Autodesk Inventor part; units mm, degrees
ref_plane "YZ Plane" through (0, 0, 0) normal (1, 0, 0) x (0, 1, 0)
ref_plane "XZ Plane" through (0, 0, 0) normal (0, 1, 0) x (-1, 0, 0)
ref_plane "XY Plane" through (0, 0, 0) normal (0, 0, 1) x (1, 0, 0)
sketch "Sketch1" plane through (0, 0, 0) normal (1, 0, 0) x (0, 1, 0)
  line L0 (0, 0) -> (25.4, 0)
  line L1 (25.4, 0) -> (25.4, -25.4)
  line L2 (25.4, -25.4) -> (0, -25.4)
  line L3 (0, -25.4) -> (0, 0)
  line L4 (23.8125, -1.5875) -> (1.5875, -1.5875)
  line L5 (1.5875, -1.5875) -> (1.5875, -23.8125)
  line L6 (1.5875, -23.8125) -> (23.8125, -23.8125)
  line L7 (23.8125, -23.8125) -> (23.8125, -1.5875)
  dimension "d0" = 25.4
  dimension "d1" = 25.4
  dimension "d2" = 1.5875
extrude "Extrusion1" add sketch "Sketch1" along normal blind 609.6
sketch "Sketch2" plane through (0, 25.4, 0) normal (0, 1, 0) x (1, 0, 0)
  line L0 (0, 1.5875) -> (0, 23.8125)
  line L1 (0, 12.7) -> (64.9449, 12.7) construction
  circle A0 centre (38.1, 12.7) radius 3.175
  circle A1 centre (63.5, 12.7) radius 3.175
  circle A2 centre (292.1, 12.7) radius 3.175
  point P0 (0, 0)
  dimension "d5" = 6.35
  dimension "d6" = 38.1
  dimension "d7" = 63.5
  dimension "d8" = 292.1
extrude "Extrusion2" cut sketch "Sketch2" against normal blind 25.4
sketch "Sketch3" plane through (0, 0, 0) normal (0, 0, 1) x (1, 0, 0)
  line L0 (0, 23.8125) -> (0, 1.5875)
  line L1 (0, 12.7) -> (84.2174, 12.7) construction
  circle A0 centre (241.3, 12.7) radius 3.175
  point P0 (0, 0)
  dimension "d11" = 6.35
  dimension "d12" = 241.3
extrude "Extrusion3" cut sketch "Sketch3" against normal blind 25.4
properties part number "Short horizontal"
Geometry: final body of the model. Coordinates: model frame, mm. A direction names the side the tool comes from. Coordinates: 2 decimals unless noted, no trailing zeros. Loops run counter-clockwise (first coordinate to the right, second up) from the corner with the lowest first, then second, coordinate; pieces in that order, holes last. Notation, with made-up numbers: (1, 72) - (6, 72) arc R7 cw to (6, 82) - close; hole circle Ø5 at (22.5, 77). An arc over 180 degrees is marked (long way). One line per question, with ' | ' between items. Start each with the question number.
(1) Draft query along Y for faces 1 (the flat face through (609.6, 1, -13)), 2 (the flat face through (301, 0, -13)), 3 (the flat face through (301, 13, -1.588)). Return one class per face: +Y half, -Y half, draft (parallel to the pull), parting line (faces both ways), or undercut.
(2) Cut plane A-A on x = 152.5. Output: boundary loops of the cut face in (y, z), and give its area (3 significant figures).
(3) Reachability of faces 4 (the flat face through (0, 1, -13)), 5 (the flat face through (301, 1.588, -13)) from +Z, -Z, +X, -X, +Y, -Y: full face, straight path, thin tool, end or side. Return the list, or none.
(4) Ray query, L1, parallel to Z at x = 63.5, y = 0.95 (3 decimals); L2, parallel to Z at x = 27.5, y = 22; L3, parallel to Y at x = 177, z = -3.5. Return the intervals inside material, ascending. Write a range as from..to.
Here are the results:
1) face 1: draft | face 2: -Y half | face 3: undercut
2) outline: (0, -25.4) - (25.4, -25.4) - (25.4, 0) - (0, 0) - close; hole (1.59, -23.81) - (23.81, -23.81) - (23.81, -1.59) - (1.59, -1.59) - close | area: 151 mm²
3) face 4: +Z, -Z, -X, +Y, -Y | face 5: +X, -X
4) L1: -25.4..-15.875, -9.525..0 | L2: -25.4..-23.81, -1.59..0 | L3: 0..1.59, 23.81..25.4
